```python
from build123d import *

# Parameters (mm, degrees)
BOSS_EXTRUDE2_DEPTH = 3
SKETCH3_W           = 80
SKETCH3_H           = 8
BOSS_EXTRUDE3_DEPTH = 2
SKETCH4_R           = 1.5
CUT_EXTRUDE5_DEPTH  = 2
SKETCH12_R          = 1.5
CUT_EXTRUDE6_DEPTH  = 2
SKETCH16_W          = 10
SKETCH16_H          = 8
CUT_EXTRUDE7_DEPTH  = 2
SKETCH17_R          = 1.5
CUT_EXTRUDE8_DEPTH  = 2
FILLET1_R           = 4


with BuildPart() as part:
    # Sketch1 → Boss-Extrude2 (new body)
    with BuildSketch(Plane(origin=(0, 0, 0), x_dir=(1, 0, 0), z_dir=(0, 1, 0))):
        with BuildLine():
            Line((-25, -4), (65, -4))
            ThreePointArc((65, -4), (69, 0), (65, 4))
            Line((65, 4), (-25, 4))
            Line((-25, 4), (-25, -4))
        make_face()
    extrude(amount=BOSS_EXTRUDE2_DEPTH)

    # Sketch3 → Boss-Extrude3 (add)
    with BuildSketch(Plane(origin=(0, 3, 0), x_dir=(1, 0, 0), z_dir=(0, 1, 0))):
        with Locations((15, 0)):
            Rectangle(SKETCH3_W, SKETCH3_H)
    extrude(amount=BOSS_EXTRUDE3_DEPTH)

    # Sketch4 → Cut-Extrude5 (cut)
    with BuildSketch(Plane(origin=(0, 3, 0), x_dir=(1, 0, 0), z_dir=(0, 1, 0))):
        with Locations(Location((65, 0, 0), (0, 0, 270))):
            Circle(SKETCH4_R)
    extrude(amount=-CUT_EXTRUDE5_DEPTH, mode=Mode.SUBTRACT)

    # Sketch12 → Cut-Extrude6 (cut)
    with BuildSketch(Plane(origin=(0, 5, 0), x_dir=(1, 0, 0), z_dir=(0, 1, 0))):
        with Locations(Location((47, 0, 0), (0, 0, 270))):
            Circle(SKETCH12_R)
        with Locations(Location((27, 0, 0), (0, 0, 270))):
            Circle(SKETCH12_R)
        with Locations(Location((7, 0, 0), (0, 0, 270))):
            Circle(SKETCH12_R)
    extrude(amount=-CUT_EXTRUDE6_DEPTH, mode=Mode.SUBTRACT)

    # Sketch16 → Cut-Extrude7 (cut)
    with BuildSketch(Plane(origin=(0, 5, 0), x_dir=(1, 0, 0), z_dir=(0, 1, 0))):
        with Locations((-20, 0)):
            Rectangle(SKETCH16_W, SKETCH16_H)
    extrude(amount=-CUT_EXTRUDE7_DEPTH, mode=Mode.SUBTRACT)

    # Sketch17 → Cut-Extrude8 (cut)
    with BuildSketch(Plane(origin=(0, 3, 0), x_dir=(1, 0, 0), z_dir=(0, 1, 0))):
        with Locations(Location((-22, 0, 0), (0, 0, 270))):
            Circle(SKETCH17_R)
    extrude(amount=-CUT_EXTRUDE8_DEPTH, mode=Mode.SUBTRACT)

    # Fillet1
    fillet1_edges = [part.edges().sort_by_distance(p)[0] for p in [
        (-25, 1.5, -4),
        (-25, 1.5, 4),
    ]]
    fillet(fillet1_edges, radius=FILLET1_R - 0.0001)  # a hair under: the kernel refuses the full size


solid = part.part
```
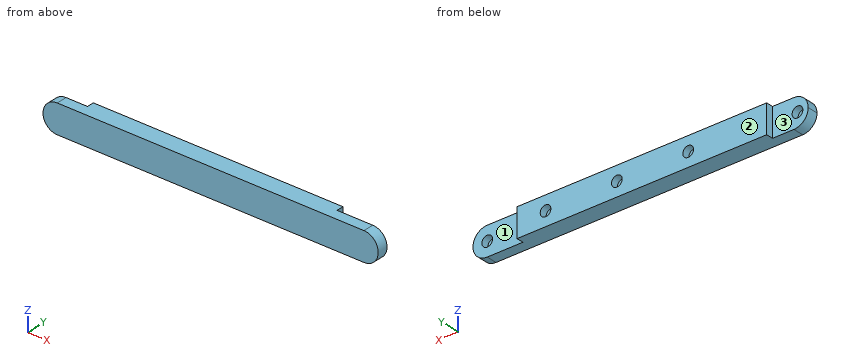
Could you check a few things on this model? Use its own coordinates, in mm. Face numbers are marked on the shaded views. A direction names the side the tool comes from. Give positions to 0.01 mm unless a question says otherwise; leave off trailing zeros. Loops run counter-clockwise (first coordinate to the right, second up) from the corner with the lowest first, then second, coordinate; pieces in that order, holes last. Notation, with made-up numbers: (-14.5, 87.5) - (29.5, 87.5) arc R26 cw to (29.5, 103.5) - close; hole circle Ø2 at (35.25, 84.5). An arc over 180 degrees is marked (long way). Use one line per item in the form item = value.
1. I need wall thicknesses on probe 1 along X at (y, z) = (4.05, 0); probe 2 along X at (y, z) = (4.05, -0.75); probe 3 along X at (y, z) = (2.9, -0.25). Which ranges of each line are inside material? Lowest first, please.
Response values:
probe_1 = -15 to 5.5, 8.5 to 25.5, 28.5 to 45.5, 48.5 to 55
probe_2 = -15 to 5.7, 8.3 to 25.7, 28.3 to 45.7, 48.3 to 55
probe_3 = -24.99 to -23.48, -20.52 to 63.52, 66.48 to 68.99
2. I want a section at B-B (z = -2.5). Please give me the cut outline in (x, y), and give its area (3 significant figures).
Response values:
outline = (-24.12, 0) - (68.12, 0) - (68.12, 3) - (55, 3) - (55, 5) - (-15, 5) - (-15, 3) - (-24.12, 3) - close
area = 417 mm²
3. I'm going to push flat-ended pins straight in: pin 1 Ø0.9 at (x, z) = (65.5, -0.5) entering from +Y; pin 2 Ø0.6 at (y, z) = (4.5, -0.5) entering from +X; pin 3 Ø0.6 at (y, z) = (3.5, -0.5) entering from -X. Where does each tip first touch, or does it pass through?
Response values:
pin_1 = 1
pin_2 = 55
pin_3 = -15
4. I want a section at A-A (x = 47). Please give me the cut outline in (y, z).
Response values:
outline = (0, -4) - (5, -4) - (5, -1.5) - (3, -1.5) - (3, 1.5) - (5, 1.5) - (5, 4) - (0, 4) - close
5. On a 3-axis mill with a long thin cutter (end or side, diameter ignored), from which of +Z, -Z, +X, -X, +Y, -Y can I reach the whole of each face in a straight line? I mean the marked faces 1, 2 and 3. Say none if no direction works.
Response values:
face_1 = +Z, -Z, +X, +Y
face_2 = +Z, -Z, +X, -X, +Y
face_3 = +Z, -Z, -X, +Y
